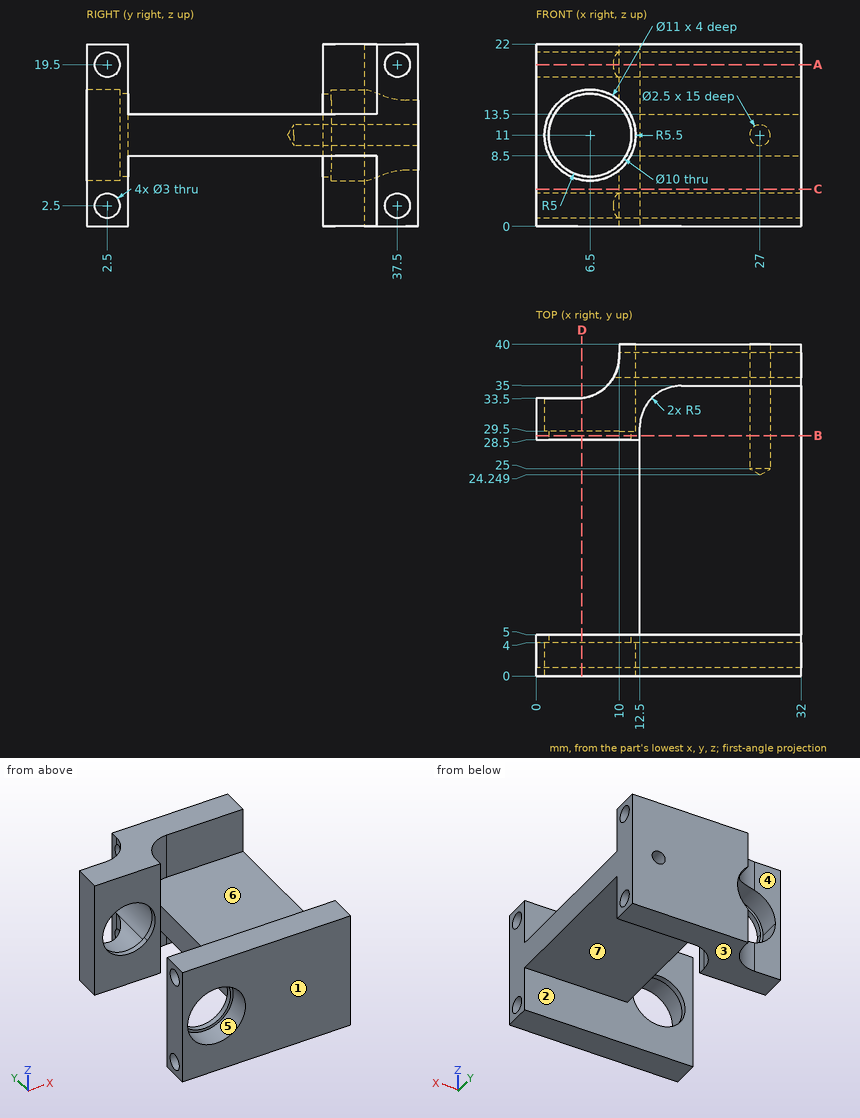
Can you work these out from the drawing? Everything is in mm from the part's minimum corner. A direction names the side the tool comes from. Coordinates: 2 decimals unless noted, no trailing zeros. Loops run counter-clockwise (first coordinate to the right, second up) from the corner with the lowest first, then second, coordinate; pieces in that order, holes last.
1) Imagine slicing it at A-A on z = 19.5. List the corners of the cut face in (x, y) for me, plus the area to 3 significant figures.
2) Imagine slicing it at B-B on y = 29. List the corners of the cut face in (x, z) for me.
3) Imagine slicing it at C-C on z = 4.5. List the corners of the cut face in (x, y) for me, plus the area to 3 significant figures.
4) For pin 1 (6.5 mm diameter, centred on x = 6.5, z = 11, fed in from -Y); pin 2 (6 mm diameter, centred on x = 20.5, y = 13, fed in from +Z); pin 3 (10 mm diameter, centred on x = 21.5, y = 19, fed in from -Z); pin 4 (5.5 mm diameter, centred on y = 13.5, z = 12, fed in from -X), each with a flat end and sliding along its axis, tell me the tip position at first contact or that it passes through.
5) Thinking about a two-plate mould opening in Y: for the marked faces 1, 2, 3 and 4, which applies, pulls with the +Y half, pulls with the -Y half, needs draft (parallel to the pull), parting line crosses it, or undercut?
6) Imagine slicing it at D-D on x = 5.5. List the corners of the cut face in (y, z) for me (3 decimals), plus the area to 3 significant figures.
7) Which directions (+Z, -Z, +X, -X, +Y, -Y) give clear straight access to the entire face, cutting with the end or side of a thin tool? Please do the marked faces 5, 6 and 7.
8) I need wall thicknesses on probe 1 along Z at (x, y) = (17, 37.5); probe 2 along Z at (x, y) = (6.5, 3); probe 3 along Y at (x, z) = (31, 14.75). Which ranges of each line are inside material? Lowest first, please.
Completed:
1. outline: (0, 0) - (32, 0) - (32, 1) - (0, 1) - close; (0, 4) - (32, 4) - (32, 5) - (0, 5) - close; (0, 28.5) - (12.5, 28.5) - (12.5, 30) arc R5 cw to (17.5, 35) - (32, 35) - (32, 36) - (9.33, 36) arc R5 cw to (5, 33.5) - (0, 33.5) - close; (10, 39) - (32, 39) - (32, 40) - (10, 40) - close
1. area: 184 mm2
2. outline: (0, 0) - (12.5, 0) - (12.5, 8.5) - (32, 8.5) - (32, 13.5) - (12.5, 13.5) - (12.5, 22) - (0, 22) - close; hole circle Ø10 at (6.5, 11); hole circle Ø2.5 at (27, 11)
3. outline: (0, 0) - (32, 0) - (32, 5) - (0, 5) - close; (0, 28.5) - (12.5, 28.5) - (12.5, 30) arc R5 cw to (17.5, 35) - (32, 35) - (32, 40) - (10, 40) - (10, 38.5) arc R5 cw to (5, 33.5) - (0, 33.5) - close
3. area: 347 mm2
4. pin 1: passes through
4. pin 2: stops at z = 13.5
4. pin 3: stops at z = 8.5
4. pin 4: stops at x = 12.5
5. face 1: pulls with the -Y half
5. face 2: undercut
5. face 3: needs draft
5. face 4: pulls with the +Y half
6. outline: (0, 0) - (5, 0) - (5, 6.101) - (4, 6.101) - (4, 5.592) - (0, 5.592) - close; (0, 16.408) - (4, 16.408) - (4, 15.899) - (5, 15.899) - (5, 22) - (0, 22) - close; (28.5, 0) - (33.525, 0) - (33.525, 5.592) - (29.5, 5.592) - (29.5, 6.101) - (28.5, 6.101) - close; (28.5, 15.899) - (29.5, 15.899) - (29.5, 16.408) - (33.525, 16.408) - (33.525, 22) - (28.5, 22) - close; hole circle Ø3 at (2.5, 2.5); hole circle Ø3 at (2.5, 19.5)
6. area: 100 mm2
7. face 5: -Y
7. face 6: +Z, +X
7. face 7: -Z, +X
8. probe 1: z = 0 to 1, 4 to 18, 21 to 22
8. probe 2: z = 0 to 1.09, 3.91 to 5.5, 16.5 to 18.09, 20.91 to 22
8. probe 3: y = 0 to 5, 35 to 40
